```python
from build123d import *

# Parameters (mm, degrees)
F0_R     = 7.5
F1_DEPTH = 800
F2_R     = 7.5
F3_DEPTH = 100
F4_W     = 40
F4_H     = 40
F5_DEPTH = 3
F7_D     = 9


with BuildPart() as f1:
    # F0 (on Top) → F1 (new body)
    with BuildSketch(Plane.XY):
        Circle(F0_R)
    extrude(amount=F1_DEPTH)

    # F2 (on Right) → F3 (join, symmetric)
    with BuildSketch(Plane.YZ):
        with Locations((0, 800)):
            Circle(F2_R)
    extrude(amount=F3_DEPTH, both=True)

    # F4 (on Front) → F5 (join, symmetric)
    with BuildSketch(Plane.XZ):
        with Locations((20, 680)):
            Rectangle(F4_W, F4_H)
    extrude(amount=F5_DEPTH, both=True)

    # F7 (through all)
    with Locations(Plane.XZ.offset(3)):
        with Locations((23.4369317712, 680)):
            Hole(F7_D / 2)

    # F8 (on Front) → F9 (revolve, cut)
    with BuildSketch(Plane.XZ):
        Polygon((10, 17.2205080757), (0.0577350269, 0), (0.0577350269, -0.1), (10, -0.1), align=None)
    revolve(axis=Axis((0, 0, 4.9), (0, 0, 1)), mode=Mode.SUBTRACT)


solid = f1.part
```
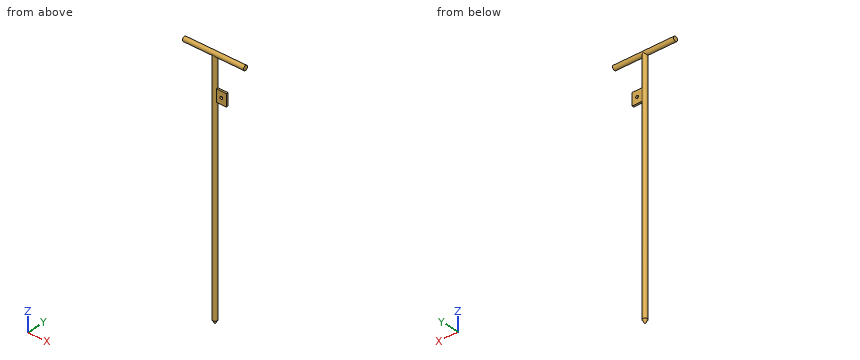
Input: part model. Units: mm. Frame: model coordinates. Give positions to 0.01 mm unless a question says otherwise; leave off trailing zeros. Write each loop counter-clockwise with the first axis right and the second up, starting at its lowest first coordinate (ties: lowest second). Pieces come first, ordered by that corner, then holes. Notation, with made-up numbers: (-29, 86) - (12, 86) arc R26 cw to (12, 112) - close; hole circle Ø7 at (9.5, -32). An arc over 180 degrees is marked (long way). Write item = value, one per line. Start each with the question number.
1) Pin query (flat end, axial travel): pin 1 (8 mm diameter, centred on x = 12.5, z = 569.5, fed in from +Y); pin 2 (4 mm diameter, centred on y = 4.5, z = 160.5, fed in from -X); pin 3 (6.5 mm diameter, centred on y = -1, z = 687, fed in from +X); pin 4 (10 mm diameter, centred on x = 19, z = 683, fed in from -Y). Return the tip coordinate at first contact, or that it passes through.
2) Cut plane A-A (z = 141). Return loops of the section in (x, y), and give its area (3 significant figures).
3) Material intervals for L1, parallel to X at y = -1.45, z = 680; L2, parallel to X at y = 0.15, z = 680; L3, parallel to Z at x = 13, y = 0, sorted ascending. Write a range as [from, to].
Answers follow:
q1.pin_1 = through
q1.pin_2 = -7.07
q1.pin_3 = 40
q1.pin_4 = -3
q2.outline = circle Ø15 at (0, 0)
q2.area = 177 mm^2
q3.L1 = [-7.36, 18.94], [27.94, 40]
q3.L2 = [-7.5, 18.94], [27.94, 40]
q3.L3 = [660, 700], [792.5, 807.5]
